The listing builds one solid part. Answer for the finished solid, in the listing's coordinates (mm). A direction names the side the tool comes from. Give positions to 0.01 mm unless a question says otherwise; leave off trailing zeros. Loops run counter-clockwise (first coordinate to the right, second up) from the corner with the lowest first, then second, coordinate; pieces in that order, holes last. Notation, with made-up numbers: M -10,-23.5 L 21,-23.5 A18 cw 21,1.5 Z; hole C 12.5,20 d1. An arc over 180 degrees is marked long. One line per item, written item: value. Start each with the question number.
Q1. A flat-ended cylindrical pin translates along its axis: pin 1 (1 mm diameter, centred on x = -19.5, y = -30.5, fed in from -Z). Find the tip coordinate at first contact, or state that the pin passes through.
Q2. A cutting plane is placed at D-D, the plane y = -36.5. Determine the outline of the cut face in (x, z).
Q3. Consider L1, parallel to X at y = 32, z = -30; L2, parallel to Y at x = 16, z = -36; L3, parallel to Y at x = 24.5, z = -65. Determine where each line is inside the solid, lowest interval first.
Q4. A cutting plane is placed at B-B, the plane x = 70.5. Determine the outline of the cut face in (y, z).
Q5. The mould has two halves that part along X. Classify faces 3 (the flat face through (19, 61.934, -38)), 4 (the flat face through (17, 58.934, -65)), 5 (the flat face through (18.1, 57.3, -50)): +X half, -X half, draft (parallel to the pull), parting line (faces both ways), or undercut.
Q6. A cutting plane is placed at A-A, the plane z = -20. Determine the outline of the cut face in (x, y), and give its area (3 significant figures).
Q7. For faces 1 (the flat face through (92, 9, -80)), 2 (the flat face through (50, 56.934, -25)), determine the directions among +Z, -Z, +X, -X, +Y, -Y from which every point of the face is accessible in a straight line to the end or side of a thin tool.
Q8. A cutting plane is placed at C-C, the plane z = -66.5. Determine the outline of the cut face in (x, y), and give its area (3 significant figures).
Autodesk Inventor part; units mm, degrees
ref_plane "YZ Plane" through (0, 0, 0) normal (1, 0, 0) x (0, 1, 0)
ref_plane "XZ Plane" through (0, 0, 0) normal (0, 1, 0) x (-1, 0, 0)
ref_plane "XY Plane" through (0, 0, 0) normal (0, 0, 1) x (1, 0, 0)
sketch "Sketch1" plane through (0, 0, 0) normal (0, 0, 1) x (1, 0, 0)
  line L0 (-51.5843, -39.0663) -> (88.4157, -39.0663)
  line L1 (88.4157, -39.0663) -> (88.4157, -9.0663)
  line L2 (88.4157, -9.0663) -> (-51.5843, -9.0663)
  line L3 (-51.5843, -9.0663) -> (-51.5843, -39.0663)
  line L4 (-53.5843, -41.0663) -> (90.4157, -41.0663)
  line L5 (90.4157, -41.0663) -> (90.4157, -7.0663)
  line L6 (90.4157, -7.0663) -> (-53.5843, -7.0663)
  line L7 (-53.5843, -7.0663) -> (-53.5843, -41.0663)
  line L8 (10.4157, -7.0663) -> (88.4157, -7.0663)
  line L9 (88.4157, -7.0663) -> (88.4157, 56.9337)
  line L10 (88.4157, 56.9337) -> (10.4157, 56.9337)
  line L11 (10.4157, 56.9337) -> (10.4157, -7.0663)
  line L12 (90.4157, 58.9337) -> (90.4157, -9.0663)
  line L13 (90.4157, -9.0663) -> (8.4157, -9.0663)
  line L14 (8.4157, -9.0663) -> (8.4157, 58.9337)
  line L15 (8.4157, 58.9337) -> (90.4157, 58.9337)
  line L16 (-53.5843, -7.0663) -> (8.4157, -7.0663)
  line L17 (8.4157, -7.0663) -> (8.4157, 58.9337)
  line L18 (8.4157, 58.9337) -> (-53.5843, 58.9337)
  line L19 (-53.5843, 58.9337) -> (-53.5843, -7.0663)
  line L20 (-51.5843, -6.0663) -> (-51.5843, 56.9337)
  line L21 (-51.5843, 56.9337) -> (9.4157, 56.9337)
  line L22 (-56.5843, -44.0663) -> (93.4157, -44.0663)
  line L23 (93.4157, -44.0663) -> (93.4157, 61.9337)
  line L24 (93.4157, 61.9337) -> (-56.5843, 61.9337)
  line L25 (-56.5843, 61.9337) -> (-56.5843, -44.0663)
  line L26 (-51.5843, -6.0663) -> (-51.5843, -9.0663)
  point P0 (0, 0)
  point P1 (90.4157, -7.0663)
  point P2 (88.4157, -7.0663)
  point P3 (10.4157, -7.0663)
  point P4 (8.4157, -7.0663)
  point P5 (-47.5843, -6.0663)
  point P6 (8.4157, 56.9337)
  point P7 (90.4157, -7.0663)
  point P8 (-51.5843, -7.0663)
  dimension "d0" = 140
  dimension "d1" = 30
  dimension "d2" = 2
  dimension "d3" = 78
  dimension "d4" = 64
  dimension "d5" = 2
  dimension "d7" = 0
  dimension "d8" = 0
  dimension "d9" = 2
  dimension "d10" = 3
  dimension "d11" = 3
  dimension "d12" = 3
  dimension "d13" = 3
extrude "Extrusion1" add sketch "Sketch1" along normal blind 3 contours L3 L2 L1 L0 | L0 L1 L13 L5 L4 L7 L6 L26 L3 | L26 L6 L14 L2 | L2 L14 L6 L5 L13 | L26 L20 L21 L14 L6 | L6 L19 L18 L14 L21 L20 L26 | L14 L15 L12 L6 L9 L10 L11 | L11 L10 L9 L6 | L25 L24 L23 L22
extrude "Extrusion2" add sketch "Sketch1" against normal blind 80
extrude "Extrusion3" add sketch "Sketch1" against normal blind 50 contours L0 L1 L13 L5 L4 L7 L6 L26 L3 | L26 L6 L14 L2 | L2 L14 L6 L5 L13 | L6 L19 L18 L14 L21 L20 L26 | L14 L15 L12 L6 L9 L10 L11
extrude "Extrusion4" add sketch "Sketch1" against normal blind 1 contours L3 L2 L1 L0 | L0 L1 L13 L5 L4 L7 L6 L26 L3 | L26 L6 L14 L2 | L2 L14 L6 L5 L13 | L26 L20 L21 L14 L6 | L6 L19 L18 L14 L21 L20 L26 | L14 L15 L12 L6 L9 L10 L11 | L11 L10 L9 L6
fillet "Fillet1" radius 2 4 edges at (93.4157, -44.0663, -38.5) (-56.5843, -44.0663, -38.5) (-56.5843, 61.9337, -38.5) (93.4157, 61.9337, -38.5)
sketch "Sketch3" plane through (-54.5843, 61.9337, -80) normal (0, 1, 0) x (1, 0, 0)
  line L0 (-2, 0) -> (0, 0)
  line L1 (-2, 0) -> (73, 0)
  line L2 (145, 0) -> (1, 0)
  circle A0 centre (73, 0) radius 2.5
  line L3 (73, 0) -> (73, -2.5)
  line L4 (73, -2.5) -> (87.7902, 0)
  line L5 (73, -2.5) -> (58.2098, 0)
  point P0 (54.5843, -80)
  point P1 (72.1783, -2.3611)
  point P2 (73.8217, -2.3611)
  point P3 (75.5, 0)
  point P4 (70.5, 0)
  dimension "d26" = 5
  dimension "d25" = 75
  dimension "d27" = 15
  dimension "d28" = 15
extrude "Extrusion6" cut sketch "Sketch3" against normal through all
fillet "Fillet2" radius 10 2 edges at (17.5941, 60.4337, -77.6389) (19.2374, 60.4337, -77.6389)
properties part number "box_kit" material "LCP Plastic"
Answer block:
1. pin 1: z = -1
2. outline: M -56.58,-80 L -53.58,-80 L -53.58,-50 L -51.58,-50 L -51.58,-1 L 88.42,-1 L 88.42,-50 L 90.42,-50 L 90.42,-80 L 93.42,-80 L 93.42,3 L -56.58,3 Z
3. L1: -56.58 to -51.58, 8.42 to 10.42, 88.42 to 93.42
3. L2: -44.07 to -39.07, -9.07 to -7.07, 56.93 to 61.93
3. L3: -44.07 to -41.07, 58.93 to 61.93
4. outline: M -44.07,-80 L -41.07,-80 L -41.07,-50 L -39.07,-50 L -39.07,-1 L -9.07,-1 L -9.07,-50 L -7.07,-50 L -7.07,-1 L 56.93,-1 L 56.93,-50 L 58.93,-50 L 58.93,-80 L 61.93,-80 L 61.93,3 L -44.07,3 Z
5. face 3: draft
5. face 4: undercut
5. face 5: undercut
6. outline: M -56.58,-42.07 A2 ccw -54.58,-44.07 L 91.42,-44.07 A2 ccw 93.42,-42.07 L 93.42,59.93 A2 ccw 91.42,61.93 L -54.58,61.93 A2 ccw -56.58,59.93 Z; hole M -51.58,-39.07 L 88.42,-39.07 L 88.42,-9.07 L -51.58,-9.07 Z; hole M -51.58,-7.07 L 8.42,-7.07 L 8.42,56.93 L -51.58,56.93 Z; hole M 10.42,-7.07 L 88.42,-7.07 L 88.42,56.93 L 10.42,56.93 Z
6. area: 2,860 mm^2
7. face 1: -Z, +X, -X, +Y, -Y
7. face 2: -Z
8. outline: M -56.58,-42.07 A2 ccw -54.58,-44.07 L 91.42,-44.07 A2 ccw 93.42,-42.07 L 93.42,59.93 A2 ccw 91.42,61.93 L -54.58,61.93 A2 ccw -56.58,59.93 Z; hole M -53.58,-41.07 L 90.42,-41.07 L 90.42,58.93 L -53.58,58.93 Z
8. area: 1,500 mm^2
